For this review, take the finished solid that the model builds, in its own axes (mm). A direction names the side the tool comes from. Give positions to 0.01 mm unless a question says otherwise; leave off trailing zeros. Loops run counter-clockwise (first coordinate to the right, second up) from the corner with the lowest first, then second, coordinate; pieces in that order, holes last. Notation, with made-up numbers: (-12.75, -34) -> (46.25, -34) arc R10 cw to (46.25, -27) -> close; hole circle Ø6 at (34, 13.5). An arc over 180 degrees is marked (long way). One line per question, with ' | ' between items. Start each with the question number.
(1) Consider section B-B (x = -1.25). Write out the cut boundary in (y, z), and give its area (3 significant figures).
(2) Consider section A-A (y = 110). Write out the cut boundary in (x, z).
(3) Tool access review of faces 5 (the flat face through (-7.5, -153, 0)), 6 (the flat face through (0, 125, 0)), 7 (the flat face through (-11, 155, 0)), 8 (the flat face through (-7.5, 152, 0)), 9 (the flat face through (0, 2, -2.5)): name each direction out of +Z, -Z, +X, -X, +Y, -Y from which nothing blocks a thin tool from reaching the whole face with its end or side.
(4) Wall thickness on probe 1 along Y at (x, z) = (2, 0.1); probe 2 along X at (y, z) = (-103, 1.6); probe 3 along Y at (x, z) = (-7, -1.95): over which ranges is each line inside the solid? List them lowest first.
(5) Consider section C-C (z = 1.05). Write out the cut boundary in (x, y).
(6) Insertion check: P1, Ø1.5, axis at x = 3, z = 1, coming from the +Y side; P2, Ø2, axis at x = -5.5, z = 0, coming from the -Y side. Each pin has a flat end and moves straight along its axis. Give the tip position at first contact, or say it passes through.
(7) Draft analysis for pull direction X (two halves, no side actions). For faces 1 (the flat face through (0, 150, 0)), 2 (the flat face through (15, -2, 0)), 3 (the flat face through (11, -155, 0)), 4 (the flat face through (7.5, -153, 0)), state which applies: +X half, -X half, draft (parallel to the pull), parting line (faces both ways), or undercut.
from build123d import *

# Parameters (mm, degrees)
F0_W     = 7.5
F0_H     = 5
F1_DEPTH = 2.5
F2_W     = 10
F2_H     = 50
F3_DEPTH = 10
F4_W     = 10
F4_H     = 50
F5_DEPTH = 10


with BuildPart() as f1:
    # F0 (on Top) → F1 (new body, symmetric)
    with BuildSketch(Plane.XY):
        Polygon((7.5, -150), (15, -150), (15, 150), (7.5, 150), (-7.5, 150), (-15, 150), (-15, -150), (-7.5, -150), align=None)
        with Locations((-11.25, -152.5)):
            Rectangle(F0_W, F0_H)
        with Locations((11.25, 152.5)):
            Rectangle(F0_W, F0_H)
        with Locations((-11.25, 152.5)):
            Rectangle(F0_W, F0_H)
        with Locations((11.25, -152.5)):
            Rectangle(F0_W, F0_H)
    extrude(amount=F1_DEPTH, both=True)

    # F2 (on face) → F3 (cut)
    with BuildSketch(Plane.XY.offset(2.5)):
        with Locations((0, -100)):
            Rectangle(F2_W, F2_H)
    extrude(amount=-F3_DEPTH, mode=Mode.SUBTRACT)

    # F4 (on face) → F5 (cut)
    with BuildSketch(Plane.XY.offset(2.5)):
        with Locations((0, 100)):
            Rectangle(F4_W, F4_H)
    extrude(amount=-F5_DEPTH, mode=Mode.SUBTRACT)


solid = f1.part
A:
1) outline: (-150, -2.5) -> (-125, -2.5) -> (-125, 2.5) -> (-150, 2.5) -> close; (-75, -2.5) -> (75, -2.5) -> (75, 2.5) -> (-75, 2.5) -> close; (125, -2.5) -> (150, -2.5) -> (150, 2.5) -> (125, 2.5) -> close | area: 1,000 mm^2
2) outline: (-15, -2.5) -> (-5, -2.5) -> (-5, 2.5) -> (-15, 2.5) -> close; (5, -2.5) -> (15, -2.5) -> (15, 2.5) -> (5, 2.5) -> close
3) face 5: +Z, -Z, -Y | face 6: +Z, -Z | face 7: +Z, -Z, +X, -X, +Y | face 8: +Z, -Z, +Y | face 9: -Z, +X, -X, +Y, -Y
4) probe 1: y = -150 to -125, -75 to 75, 125 to 150 | probe 2: x = -15 to -5, 5 to 15 | probe 3: y = -150 to 150
5) outline: (-15, -155) -> (-7.5, -155) -> (-7.5, -150) -> (7.5, -150) -> (7.5, -155) -> (15, -155) -> (15, 155) -> (7.5, 155) -> (7.5, 150) -> (-7.5, 150) -> (-7.5, 155) -> (-15, 155) -> close; hole (-5, -125) -> (5, -125) -> (5, -75) -> (-5, -75) -> close; hole (-5, 75) -> (5, 75) -> (5, 125) -> (-5, 125) -> close
6) P1: stops at y = 150 | P2: stops at y = -150
7) face 1: undercut | face 2: +X half | face 3: draft | face 4: undercut
